from build123d import *

# Parameters (mm, degrees)
SKETCH1_W                                        = 152.4
SKETCH1_H                                        = 152.4
BOSS_EXTRUDE1_DEPTH                              = 19.05
CBORE_FOR_1_4_SOCKET_HEAD_CAP_SCREW1_D           = 6.5278
CBORE_FOR_1_4_SOCKET_HEAD_CAP_SCREW1_CBORE_D     = 11.1125
CBORE_FOR_1_4_SOCKET_HEAD_CAP_SCREW1_CBORE_DEPTH = 8.89
T_SLOT_CUT_WITH_MCMASTER_8789A16_BIT_DEPTH       = 172.45
FILLET1_R                                        = 3.175


with BuildPart() as part:
    # Sketch1 → Boss-Extrude1 (new body)
    with BuildSketch(Plane(origin=(0, 0, 0), x_dir=(1, 0, 0), z_dir=(0, 1, 0))):
        Rectangle(SKETCH1_W, SKETCH1_H)
    extrude(amount=BOSS_EXTRUDE1_DEPTH)

    # CBORE for 1/4 Socket Head Cap Screw1 (through all)
    with Locations(Plane(origin=(0, 19.05, 0), x_dir=(1, 0, 0), z_dir=(0, 1, 0))):
        with Locations((-63.5, 63.5), (63.5, 63.5), (63.5, -63.5), (-63.5, -63.5)):
            CounterBoreHole(CBORE_FOR_1_4_SOCKET_HEAD_CAP_SCREW1_D / 2, CBORE_FOR_1_4_SOCKET_HEAD_CAP_SCREW1_CBORE_D / 2, CBORE_FOR_1_4_SOCKET_HEAD_CAP_SCREW1_CBORE_DEPTH)

    # Sketch4 → T-SLOT CUT WITH MCMASTER 8789A16 BIT (cut, through all)
    with BuildSketch(Plane(origin=(-76.2, 0, 0), x_dir=(0, 0, -1), z_dir=(1, 0, 0))):
        Polygon((-40.8765375, 19.05), (-40.8765375, 12.7), (-44.64685, 12.7), (-44.64685, 6.746875), (-30.35935, 6.746875), (-30.35935, 12.7), (-34.1296625, 12.7), (-34.1296625, 19.05), align=None)
        Polygon((34.1296625, 12.7), (34.1296625, 19.05), (40.8765375, 19.05), (40.8765375, 12.7), (44.64685, 12.7), (44.64685, 6.746875), (30.35935, 6.746875), (30.35935, 12.7), align=None)
    extrude(amount=T_SLOT_CUT_WITH_MCMASTER_8789A16_BIT_DEPTH, mode=Mode.SUBTRACT)

    # Fillet1
    fillet1_edges = [part.edges().sort_by_distance(p)[0] for p in [
        (76.2, 9.525, 76.2),
        (-76.2, 9.525, 76.2),
        (-76.2, 9.525, -76.2),
        (76.2, 9.525, -76.2),
    ]]
    fillet(fillet1_edges, radius=FILLET1_R)


solid = part.part
Check sheet for the modelled part. Datum: model origin and axes. Units: mm. A direction names the side the tool comes from. Give positions to 0.01 mm unless a question says otherwise; leave off trailing zeros. Loops run counter-clockwise (first coordinate to the right, second up) from the corner with the lowest first, then second, coordinate; pieces in that order, holes last. Notation, with made-up numbers: M 3,-40 L 57,-40 A20 ccw 57,-14 Z; hole C 87.25,-21 d1. An arc over 180 degrees is marked long. Use a Markdown table: item, result. Add a question column.
Q1. Tool access check on faces 1 (the flat face through (-61, 10.16, -61)), 2 (the flat face through (-1, 0, -1)), 3 (the cylindrical face through (61.745, 5.009, -66.252)), 4 (the flat face through (-1, 10, 30.359)), 5 (the flat face through (-1, 16, -40.877)). Record the directions out of +Z, -Z, +X, -X, +Y, -Y that give a thin tool (end or side, any length) a straight path to the whole face; none if there is none.
Q2. Mould release check, pull along X, two halves, no side actions. Record for faces 6 (the flat face through (66, 10.16, 66)), 7 (the flat face through (76.2, 9, 1)), 8 (the flat face through (-1, 12.7, -43)): pulls with the +X half, pulls with the -X half, needs draft (parallel to the pull), parting line crosses it, or undercut.
Q3. Go/stop test with flat-tipped pins: pin 1 (5 mm diameter, centred on x = -63.5, z = 63.5, fed in from -Y); pin 2 (3.5 mm diameter, centred on x = -66, z = -63, fed in from +Y). Record where each tip stops, or that it passes through.
Q4. Sectioned sample at C-C, the plane x = 26. Record the cut outline in (y, z).
Q5. Scan lines: line 1 along Z through (x, y) = (-63.5, 15.5); line 2 along X through (y, z) = (6.5, -63.5); line 3 along Z through (x, y) = (17.5, 11.75). Record each from-to range of solid material in increasing order. Write a range as [from, to].
Q6. Sectioned sample at B-B, the plane z = -63.5. Record the cut outline in (x, y), then the cut area to 3 significant figures.
Q7. Sectioned sample at A-A, the plane y = 17. Give the number of separate pieces and of enclosed holes in the cut face, then the cut area to 3 significant figures.
Verdict:
| question | item | result |
|---|---|---|
| 1 | face 1 | +Y |
| 1 | face 2 | +Z, -Z, +X, -X, -Y |
| 1 | face 3 | +Y, -Y |
| 1 | face 4 | +X, -X |
| 1 | face 5 | +X, -X, +Y |
| 2 | face 6 | undercut |
| 2 | face 7 | pulls with the +X half |
| 2 | face 8 | needs draft |
| 3 | pin 1 | through |
| 3 | pin 2 | y = 10.16 |
| 4 | outline | M 0,-76.2 L 19.05,-76.2 L 19.05,-40.88 L 12.7,-40.88 L 12.7,-44.65 L 6.75,-44.65 L 6.75,-30.36 L 12.7,-30.36 L 12.7,-34.13 L 19.05,-34.13 L 19.05,34.13 L 12.7,34.13 L 12.7,30.36 L 6.75,30.36 L 6.75,44.65 L 12.7,44.65 L 12.7,40.88 L 19.05,40.88 L 19.05,76.2 L 0,76.2 Z |
| 5 | line 1 | [-76.2, -69.06], [-57.94, -40.88], [-34.13, 34.13], [40.88, 57.94], [69.06, 76.2] |
| 5 | line 2 | [-76.2, -66.76], [-60.24, 60.24], [66.76, 76.2] |
| 5 | line 3 | [-76.2, -44.65], [-30.36, 30.36], [44.65, 76.2] |
| 6 | outline | M -76.2,0 L -66.76,0 L -66.76,10.16 L -69.06,10.16 L -69.06,19.05 L -76.2,19.05 Z; M -60.24,0 L 60.24,0 L 60.24,10.16 L 57.94,10.16 L 57.94,19.05 L -57.94,19.05 L -57.94,10.16 L -60.24,10.16 Z; M 66.76,0 L 76.2,0 L 76.2,19.05 L 69.06,19.05 L 69.06,10.16 L 66.76,10.16 Z |
| 6 | area | 2,570 mm^2 |
| 7 | separate pieces | 3 |
| 7 | enclosed holes | 4 |
| 7 | area | 20,800 mm^2 |
